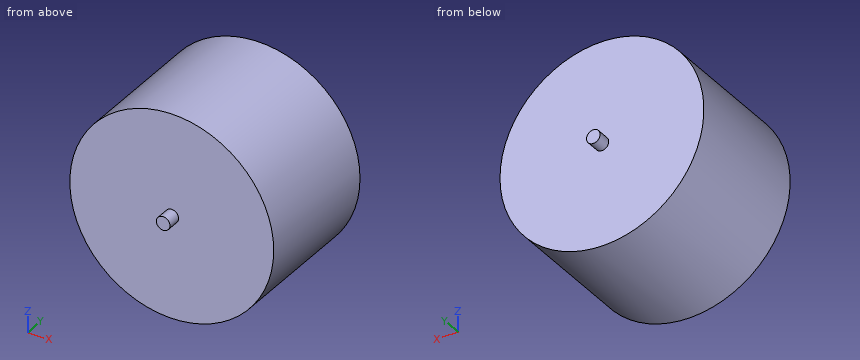
Solid Edge part; units mm, degrees
sketch "Sketch1" plane through (0, 0, 0) normal (0, -1, 0) x (1, 0, 0)
  circle A0 centre (-47.8251, 6.7192) radius 75
extrude "Protrusion1" add sketch "Sketch1" against normal blind 100
sketch "Sketch2" plane through (-47.8251, 0, 6.7192) normal (0, -1, 0) x (1, 0, 0)
  circle A0 centre (0, 0) radius 5
extrude "ExtrudedProtrusion_3" add sketch "Sketch2" along normal blind 10
sketch "Sketch3" plane through (-47.8251, 100, 6.7192) normal (0, 1, 0) x (-1, 0, 0)
  circle A0 centre (0, 0) radius 5
extrude "ExtrudedProtrusion_4" add sketch "Sketch3" along normal blind 10
CAD build for the part. Positions are in the model's coordinates, mm. Coordinates: 2 decimals unless noted, no trailing zeros. Loops run counter-clockwise (first coordinate to the right, second up) from the corner with the lowest first, then second, coordinate; pieces in that order, holes last. Notation, with made-up numbers: (48, 26.25) -> (60, 26.25) arc R28 cw to (60, 60.25) -> close; hole circle Ø9 at (24, 50). An arc over 180 degrees is marked (long way). One line per item, written item: value.
1. Drill centre lines: line 1 (Y direction, x = -9.5, z = 23); line 2 (X direction, y = 47, z = 28); line 3 (X direction, y = 22, z = -41.5). Where is each one in solid material? Low to high. Write a range as [from, to].
Answers:
line 1: y = [0, 100]
line 2: x = [-119.74, 24.09]
line 3: x = [-105.27, 9.62]
2. Slice it at A-A on x = -61.5. Write the cut outline in (y, z), and give its area (3 significant figures).
Answers:
outline: (0, -67.02) -> (100, -67.02) -> (100, 80.46) -> (0, 80.46) -> close
area: 14,700 mm^2
3. Flat gauge pins, fed straight in: P1, Ø6, axis at x = -64, y = 49.5, coming from the -Z side; P2, Ø5, axis at x = -96.5, y = 72, coming from the +Z side; P3, Ø1, axis at x = -8.5, z = -43, coming from the +Y side. Where does each tip first touch, or does it go through?
Answers:
P1: stops at z = -67.11
P2: stops at z = 65.82
P3: stops at y = 100
4. Slice it at C-C on y = 89.5. Write the cut outline in (x, z), and give its area (3 significant figures).
Answers:
outline: circle Ø150 at (-47.83, 6.72)
area: 17,700 mm^2
5. Slice it at B-B on z = 28.5. Write the cut outline in (x, y), and give its area (3 significant figures).
Answers:
outline: (-119.59, 0) -> (23.94, 0) -> (23.94, 100) -> (-119.59, 100) -> close
area: 14,400 mm^2
